Could you check a few things on this model? Use its own coordinates, in mm. A direction names the side the tool comes from. Give positions to 0.01 mm unless a question says otherwise; leave off trailing zeros. Loops run counter-clockwise (first coordinate to the right, second up) from the corner with the lowest first, then second, coordinate; pieces in that order, holes last. Notation, with made-up numbers: (28.25, 11.25) -> (32.25, 11.25) arc R20 cw to (32.25, 20.25) -> close; hole circle Ø11 at (18, 5.25). An arc over 180 degrees is marked (long way). Put each result on its own line as item: value.
Autodesk Inventor part; units mm, degrees
ref_plane "YZ Plane" through (0, 0, 0) normal (1, 0, 0) x (0, 1, 0)
ref_plane "XZ Plane" through (0, 0, 0) normal (0, 1, 0) x (-1, 0, 0)
ref_plane "XY Plane" through (0, 0, 0) normal (0, 0, 1) x (1, 0, 0)
sketch "Sketch1" plane through (0, 0, 0) normal (0, 1, 0) x (-1, 0, 0)
  line L0 (-12.7, 25.4) -> (12.7, 25.4)
  line L1 (12.7, 25.4) -> (12.7, -25.4)
  line L2 (12.7, -25.4) -> (-12.7, -25.4)
  line L3 (-12.7, -25.4) -> (-12.7, 25.4)
  line L4 (-12.7, 25.4) -> (12.7, -25.4) construction
  line L5 (12.7, 25.4) -> (-12.7, -25.4) construction
  line L6 (11.1125, 23.8125) -> (-11.1125, 23.8125)
  line L7 (-11.1125, 23.8125) -> (-11.1125, -23.8125)
  line L8 (-11.1125, -23.8125) -> (11.1125, -23.8125)
  line L9 (11.1125, -23.8125) -> (11.1125, 23.8125)
  line L10 (11.1125, 23.8125) -> (-11.1125, -23.8125) construction
  line L11 (-11.1125, 23.8125) -> (11.1125, -23.8125) construction
  point P0 (0, 0)
  dimension "d0" = 25.4
  dimension "d1" = 50.8
  dimension "d2" = 22.225
  dimension "d3" = 47.625
extrude "Extrusion1" add sketch "Sketch1" along normal blind 254
sketch "Sketch2" plane through (12.7, 0, 25.4) normal (1, 0, 0) x (0, 0, -1)
  line L0 (0, 254) -> (50.8, 254)
  line L1 (49.2125, 0) -> (49.2125, 254)
  point P0 (25.4, 0)
  point P1 (23.8125, 228.6)
  dimension "d13" = 25.4
  dimension "d14" = 25.4
hole "Hole1" at (12.7, 228.6, 1.5875) direction (-1, 0, 0) diameter 28.575 end through all
properties part number "2x1 Top" material "Aluminum 6061"
1. If we section it at A-A (y = 228.6): List the corners of the cut face in (x, z) for me (1 decimal), then the cut area to 3 significant figures.
Recorded:
outline: (-12.7, -25.4) -> (12.7, -25.4) -> (12.7, -12.7) -> (11.1, -12.7) -> (11.1, -23.8) -> (-11.1, -23.8) -> (-11.1, -12.7) -> (-12.7, -12.7) -> close; (-12.7, 15.9) -> (-11.1, 15.9) -> (-11.1, 23.8) -> (11.1, 23.8) -> (11.1, 15.9) -> (12.7, 15.9) -> (12.7, 25.4) -> (-12.7, 25.4) -> close
area: 141 mm^2
2. Thinking about a two-plate mould opening in X: for faces 1 (the face through (0, 125, -25.4)), 2 (the face through (-12.7, 125, 0)), 3 (the face through (0, 125, 23.812)), which applies, pulls with the +X half, pulls with the -X half, needs draft (parallel to the pull), parting line crosses it, or undercut?
Recorded:
face 1: needs draft
face 2: pulls with the -X half
face 3: undercut
3. If we section it at B-B (x = 5.5): List the corners of the cut face in (y, z) for me.
Recorded:
outline: (0, -25.4) -> (254, -25.4) -> (254, -23.81) -> (0, -23.81) -> close; (0, 23.81) -> (254, 23.81) -> (254, 25.4) -> (0, 25.4) -> close
4. I need wall thicknesses on line 1 (X direction, y = 92, z = -19); line 2 (Z direction, x = -1, y = 98.5); line 3 (Z direction, x = -11.85, y = 228.6) (3 decimals). Which ranges of each line are inside material? Lowest first, please.
Recorded:
line 1: x = -12.7 to -11.11, 11.11 to 12.7
line 2: z = -25.4 to -23.81, 23.81 to 25.4
line 3: z = -25.4 to -12.7, 15.875 to 25.4
5. If we section it at D-D (y = 185): List the corners of the cut face in (x, z) for me.
Recorded:
outline: (-12.7, -25.4) -> (12.7, -25.4) -> (12.7, 25.4) -> (-12.7, 25.4) -> close; hole (-11.11, -23.81) -> (11.11, -23.81) -> (11.11, 23.81) -> (-11.11, 23.81) -> close
6. If we section it at C-C (z = 11): List the corners of the cut face in (x, y) for me, then the cut area to 3 significant figures.
Recorded:
outline: (-12.7, 0) -> (-11.11, 0) -> (-11.11, 217.85) -> (-12.7, 217.85) -> close; (-12.7, 239.35) -> (-11.11, 239.35) -> (-11.11, 254) -> (-12.7, 254) -> close; (11.11, 0) -> (12.7, 0) -> (12.7, 217.85) -> (11.11, 217.85) -> close; (11.11, 239.35) -> (12.7, 239.35) -> (12.7, 254) -> (11.11, 254) -> close
area: 738 mm^2
7. For faces 4 (the face through (0, 125, -23.812)), 5 (the face through (11.9, 242.55, 4.68)), which set-ups out of +Z, -Z, +X, -X, +Y, -Y let a thin tool reach every point of the face, with its end or its side?
Recorded:
face 4: +Y, -Y
face 5: +X, -X
